For this review, take the finished solid that the model builds, in its own axes (mm). A direction names the side the tool comes from. Round coordinates to 2 decimals unless told otherwise and drop trailing zeros. Write each loop counter-clockwise with the first axis right and the second up, starting at its lowest first coordinate (ties: lowest second). Pieces come first, ordered by that corner, then holes.
from build123d import *

# Parameters (mm, degrees)
SKETCH1_W           = 20
SKETCH1_H           = 20
BOSS_EXTRUDE1_DEPTH = 5
SKETCH2_W           = 60.136694628
SKETCH2_H           = 20
BOSS_EXTRUDE2_DEPTH = 100
SKETCH3_W           = 15
SKETCH3_H           = 2
SKETCH3_H_2         = 5
SKETCH3_H_3         = 4
BOSS_EXTRUDE3_DEPTH = 230


with BuildPart() as part:
    # Sketch1 → Boss-Extrude1 (new body)
    with BuildSketch(Plane(origin=(0, 0, 0), x_dir=(1, 0, 0), z_dir=(0, 1, 0))):
        Polygon((52.700369914, 19.481718454), (32.700369914, 19.481718454), (32.700369914, -180.518281546), (-27.299630086, -180.518281546), (-27.299630086, -200.518281546), (52.700369914, -200.518281546), align=None)
        Polygon((-27.299630086, 19.481718454), (32.700369914, 19.481718454), (52.700369914, 19.481718454), (52.700369914, 39.481718454), (-47.299630086, 39.481718454), (-47.299630086, -180.518281546), (-27.299630086, -180.518281546), align=None)
        with Locations((-37.299630086, -190.518281546)):
            Rectangle(SKETCH1_W, SKETCH1_H)
    extrude(amount=BOSS_EXTRUDE1_DEPTH)

    # Sketch2 → Boss-Extrude2 (add)
    with BuildSketch(Plane(origin=(0, 5, 0), x_dir=(1, 0, 0), z_dir=(0, 1, 0))):
        with Locations((2.768717228, 29.481718454)):
            Rectangle(SKETCH2_W, SKETCH2_H)
    extrude(amount=BOSS_EXTRUDE2_DEPTH)

    # Sketch3 → Boss-Extrude3 (add)
    with BuildSketch(Plane.XY.offset(-19.481718454)):
        with Locations((-19.799630086, 104)):
            Rectangle(SKETCH3_W, SKETCH3_H)
        with Locations((25.337064542, 102.5)):
            Rectangle(SKETCH3_W, SKETCH3_H_2)
        with Locations((5.71340039, 103)):
            Rectangle(SKETCH3_W, SKETCH3_H_3)
    extrude(amount=BOSS_EXTRUDE3_DEPTH)


solid = part.part
(1) For pin 1 Ø12 at (x, z) = (-16, 84.5) entering from -Y; pin 2 Ø1 at (x, y) = (-1, 73.5) entering from +Z; pin 3 Ø1.5 at (x, y) = (-19, 2) entering from +Z, all flat-tipped, find the tip position at first contact; note any pin that passes through.
Geometry check:
pin 1: stops at y = 103
pin 2: stops at z = -19.48
pin 3: stops at z = 200.52
(2) We need section D-D, the plane x = -38.5. Give the boundary of the cut face in (y, z), and give its area (3 significant figures).
Geometry check:
outline: (0, -39.48) - (5, -39.48) - (5, 200.52) - (0, 200.52) - close
area: 1,200 mm2
(3) We need section A-A, the plane z = 177. Give the boundary of the cut face in (x, y), and give its area (3 significant figures).
Geometry check:
outline: (-47.3, 0) - (-27.3, 0) - (-27.3, 5) - (-47.3, 5) - close; (-27.3, 103) - (-12.3, 103) - (-12.3, 105) - (-27.3, 105) - close; (-1.79, 101) - (13.21, 101) - (13.21, 105) - (-1.79, 105) - close; (17.84, 100) - (32.84, 100) - (32.84, 105) - (17.84, 105) - close; (32.7, 0) - (52.7, 0) - (52.7, 5) - (32.7, 5) - close
area: 365 mm2
(4) We need section C-C, the plane y = 60. Give the boundary of the cut face in (x, z).
Geometry check:
outline: (-27.3, -39.48) - (32.84, -39.48) - (32.84, -19.48) - (-27.3, -19.48) - close
(5) For faces 5 (the face through (2, 2, 200.518)), 6 (the face through (-27.3, 2, 82)), 7 (the face through (32.837, 103, 12)), 8 (the face through (-31, 0, 79)), 9 (the face through (25, 103, 210.518)), list the 3-axis set-ups (+Z, -Z, +X, -X, +Y, -Y) from which the entire face can be reached by the end or side of a thin tool; tool diameter is ignored.
Geometry check:
face 5: +Z, +X, -X, -Y
face 6: -Y
face 7: +Z, -Z, +X, +Y
face 8: +Z, -Z, +X, -X, -Y
face 9: +Z, +X, -X, +Y, -Y
(6) Mouldability with a two-part tool opening along X and no side actions: class faces 1 (the face through (32.7, 2, 79)), 2 (the face through (-27.3, 55, -26)), 3 (the face through (-20, 103, 94)), 4 (the face through (3, 2, 180.518)) as pulls with the +X half, pulls with the -X half, needs draft (parallel to the pull), parting line crosses it, or undercut.
Geometry check:
face 1: undercut
face 2: pulls with the -X half
face 3: needs draft
face 4: undercut
(7) We need section B-B, the plane x = -18. Give the boundary of the cut face in (y, z), and give its area (3 significant figures).
Geometry check:
outline: (0, -39.48) - (105, -39.48) - (105, 210.52) - (103, 210.52) - (103, -19.48) - (0, -19.48) - close; (0, 180.52) - (5, 180.52) - (5, 200.52) - (0, 200.52) - close
area: 2,660 mm2
(8) For line 1 along Y through (x, z) = (-22.5, 185); line 2 along Y through (x, z) = (-38, 11); line 3 along Z through (x, y) = (25, 43), list the stretches that pass through material, from the lowest coordinate up.
Geometry check:
line 1: y = 0 to 5, 103 to 105
line 2: y = 0 to 5
line 3: z = -39.48 to -19.48
